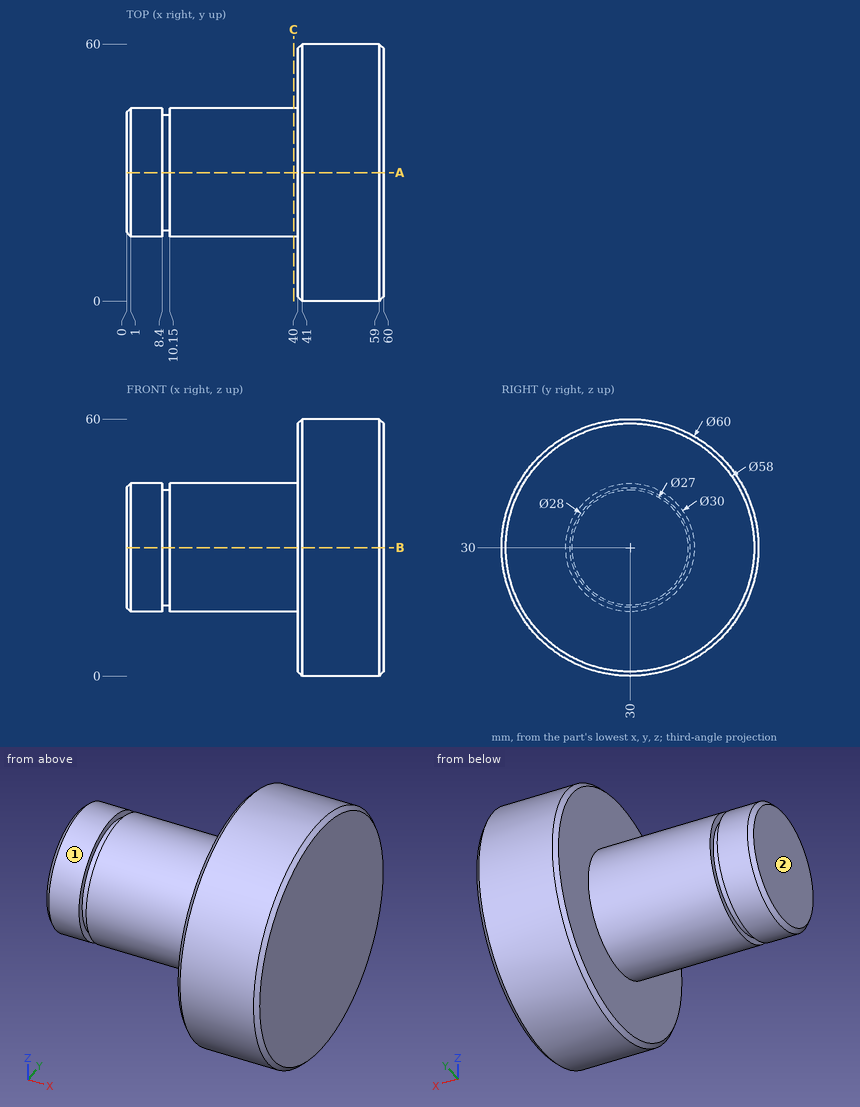
Check sheet for the drawn part. Datum: minimum x, y, z corner. Units: mm. A direction names the side the tool comes from. Round coordinates to 2 decimals unless told otherwise and drop trailing zeros. Loops run counter-clockwise (first coordinate to the right, second up) from the corner with the lowest first, then second, coordinate; pieces in that order, holes last.
Item 1: Access from +Z, -Z, +X, -X, +Y, -Y to the whole of each face (thin tool, end or side, straight path). Record for the marked faces 1 and 2.
Item 2: Thickness scan on line 1 (X direction, y = 13.5, z = 40.5); line 2 (Y direction, x = 49, z = 30); line 3 (Y direction, x = 41, z = 51). Record the ranges inside material, lowest first.
Item 3: Cross-section at C-C on x = 39. Record the boundary of the cut face in (y, z).
Item 4: Gauge pin test, flat ends, axial feed: pin 1 (6 mm diameter, centred on x = 50, z = 9, fed in from +Y); pin 2 (4 mm diameter, centred on x = 24, y = 20.5, fed in from +Z); pin 3 (1.5 mm diameter, centred on x = 22, z = 43.5, fed in from -Y). Record the tip position at first contact, or that the pin passes through.
Item 5: Cross-section at A-A on y = 30. Record the boundary of the cut face in (x, z).
Answer sheet:
1. face 1: -X
1. face 2: +Z, -Z, -X, +Y, -Y
2. line 1: x = 40 to 60
2. line 2: y = 0 to 60
2. line 3: y = 8.58 to 51.42
3. outline: circle Ø30 at (30, 30)
4. pin 1: stops at y = 54
4. pin 2: stops at z = 42.99
4. pin 3: stops at y = 22.1
5. outline: (0, 16) - (1, 15) - (8.4, 15) - (8.4, 16.5) - (10.15, 16.5) - (10.15, 15) - (40, 15) - (40, 1) - (41, 0) - (59, 0) - (60, 1) - (60, 59) - (59, 60) - (41, 60) - (40, 59) - (40, 45) - (10.15, 45) - (10.15, 43.5) - (8.4, 43.5) - (8.4, 45) - (1, 45) - (0, 44) - close
